```python
from build123d import *

# Parameters (mm, degrees)
BOSS_EXTRUDE1_DEPTH = 7
SKETCH2_R           = 3.5
BOSS_EXTRUDE2_DEPTH = 1
SKETCH3_R           = 2.5
BOSS_EXTRUDE3_DEPTH = 7


with BuildPart() as part:
    # Sketch1 → Boss-Extrude1 (new body)
    with BuildSketch(Plane.XY):
        Polygon((2.291287847, -1.026567818), (1, -1.026567818), (1, -2.317855665), (-1, -2.317855665), (-1, -1.026567818), (-2.291287847, -1.026567818), (-2.291287847, 0.973432182), (-1, 0.973432182), (-1, 2.26472003), (1, 2.26472003), (1, 0.973432182), (2.291287847, 0.973432182), align=None)
    extrude(amount=BOSS_EXTRUDE1_DEPTH)

    # Sketch2 → Boss-Extrude2 (add)
    with BuildSketch(Plane.XY.offset(7)):
        Circle(SKETCH2_R)
    extrude(amount=BOSS_EXTRUDE2_DEPTH)

    # Sketch3 → Boss-Extrude3 (add)
    with BuildSketch(Plane.XY.offset(8)):
        Circle(SKETCH3_R)
    extrude(amount=BOSS_EXTRUDE3_DEPTH)


solid = part.part
```
Model file for the job. Use its own axes, mm. A direction names the side the tool comes from. Coordinates: 2 decimals unless noted, no trailing zeros. Order: outer loops, then holes, each group sorted by start corner. A loop starts at its lowest first (then second) coordinate and runs counter-clockwise, first axis right, second up. Notation, with made-up numbers: M 42,6 L 94,6 A27 cw 94,29 Z; hole C 49,49.5 d2. An arc over 180 degrees is marked long. Answer as CSV lines item,"result".
(1) Flat gauge pins, fed straight in: pin 1 (1.4 mm diameter, centred on y = -1.5, z = 4, fed in from +X); pin 2 (0.6 mm diameter, centred on y = 2, z = 5, fed in from +X); pin 3 (4 mm diameter, centred on y = -1.5, z = 11, fed in from -X). Where does each tip first touch, or does it go through?
Geometry says:
pin 1,"stops at x = 2.29"
pin 2,"stops at x = 1"
pin 3,"stops at x = -2.5"
(2) Pull direction Y, two halves, no side cores. Call faces 1 (the cylindrical face through (3.233, -1.341, 7.493)), 2 (the flat face through (-2, -1.027, 3)), 3 (the flat face through (-2, 0.973, 3)): +Y half, -Y half, draft (parallel to the pull), parting line (faces both ways), or undercut.
Geometry says:
face 1,"parting line"
face 2,"-Y half"
face 3,"+Y half"
(3) Wall check: line 1 along X through (y, z) = (-1, 9.75); line 2 along Z through (x, y) = (-2.75, 0.5). Give the ranges that are in metal, low to high.
Geometry says:
line 1,"x = -2.29 to 2.29"
line 2,"z = 7 to 8"
(4) 3-axis set-ups, long thin cutter, end or side, ignore diameter. For faces 4 (the flat face through (0, -2.318, 3)), 5 (the flat face through (1, -2, 3)), 6 (the cylindrical face through (-0.54, -2.44, 11.45)), 7 (the flat face through (-1, -2, 3)): which of +Z, -Z, +X, -X, +Y, -Y reach the whole face in a straight line?
Geometry says:
face 4,"-Z, +X, -X, -Y"
face 5,"-Z, +X, -Y"
face 6,"+Z"
face 7,"-Z, -X, -Y"
(5) Band-saw the part on A-A, the plane y = 0. List the corners of the cut face in (x, z), then the cut area to 3 significant figures.
Geometry says:
outline,"M -3.5,7 L -2.29,7 L -2.29,0 L 2.29,0 L 2.29,7 L 3.5,7 L 3.5,8 L 2.5,8 L 2.5,15 L -2.5,15 L -2.5,8 L -3.5,8 Z"
area,"74.1 mm2"
(6) Band-saw the part on B-B, the plane z = 6.75. List the corners of the cut face in (x, y), then the cut area to 3 significant figures.
Geometry says:
outline,"M -2.29,-1.03 L -1,-1.03 L -1,-2.32 L 1,-2.32 L 1,-1.03 L 2.29,-1.03 L 2.29,0.97 L 1,0.97 L 1,2.26 L -1,2.26 L -1,0.97 L -2.29,0.97 Z"
area,"14.3 mm2"
